Read the model definition and answer for the solid it produces. Units are mm, in the model's axes. A direction names the side the tool comes from. Coordinates: 2 decimals unless noted, no trailing zeros. Loops run counter-clockwise (first coordinate to the right, second up) from the corner with the lowest first, then second, coordinate; pieces in that order, holes last.
from build123d import *

# Parameters (mm, degrees)
SKETCH1_R           = 1.675
BOSS_EXTRUDE1_DEPTH = 4
CUT_EXTRUDE1_DEPTH  = 2.5
SKETCH3_R           = 1.6
BOSS_EXTRUDE2_DEPTH = 4.5
FILLET1_R           = 0.5


with BuildPart() as part:
    # Sketch1 → Boss-Extrude1 (new body, symmetric)
    with BuildSketch(Plane.XY):
        with BuildLine():
            Line((13, -4.031128874), (17, -4.031128874))
            ThreePointArc((17, -4.031128874), (15, 4.5), (13, -4.031128874))
        make_face()
        with Locations((15, 0)):
            Circle(SKETCH1_R, mode=Mode.SUBTRACT)
    extrude(amount=BOSS_EXTRUDE1_DEPTH, both=True)

    # Sketch2 → Cut-Extrude1 (cut, symmetric)
    with BuildSketch(Plane.XY):
        with BuildLine():
            Line((11.381384933, -2.675), (18.618615067, -2.675))
            ThreePointArc((18.618615067, -2.675), (15, 4.5), (11.381384933, -2.675))
        make_face()
    extrude(amount=CUT_EXTRUDE1_DEPTH, both=True, mode=Mode.SUBTRACT)

    # Sketch3 → Boss-Extrude2 (add)
    with BuildSketch(Plane.XZ.offset(4.031128874)):
        with Locations((15, 0)):
            Circle(SKETCH3_R)
    extrude(amount=BOSS_EXTRUDE2_DEPTH)

    # Fillet1
    fillet1_edges = [part.edges().sort_by_distance(p)[0] for p in [
        (13.4, -4.031128874, 0),
    ]]
    fillet(fillet1_edges, radius=FILLET1_R)


solid = part.part
Item 1: Which of the six approach directions +Z, -Z, +X, -X, +Y, -Y give full straight-line access (tool end or side, diameter ignored) to faces 5 (the face through (15, 2, -2.5)), 6 (the face through (17.97, -3.38, 0.06))?
Numbers:
face 5: +X, -X, +Y
face 6: +Z, -Z
Item 2: A cutting plane is placed at D-D on z = 2.25. Determine the outline of the cut face in (x, y) (3 decimals), then the cut area to 3 significant figures.
Numbers:
outline: (11.381, -2.675) arc R4.5 ccw to (13, -4.031) - (17, -4.031) arc R4.5 ccw to (18.619, -2.675) - close
area: 7.97 mm2
Item 3: A cutting plane is placed at B-B on x = 15. Determine the outline of the cut face in (y, z) (3 decimals), then the cut area to 3 significant figures.
Numbers:
outline: (-8.531, -1.6) - (-4.531, -1.6) arc R0.5 cw to (-4.031, -2.1) - (-4.031, -4) - (-1.675, -4) - (-1.675, -2.5) - (-2.675, -2.5) - (-2.675, 2.5) - (-1.675, 2.5) - (-1.675, 4) - (-4.031, 4) - (-4.031, 2.1) arc R0.5 cw to (-4.531, 1.6) - (-8.531, 1.6) - close; (1.675, -4) - (4.5, -4) - (4.5, -2.5) - (1.675, -2.5) - close; (1.675, 2.5) - (4.5, 2.5) - (4.5, 4) - (1.675, 4) - close
area: 36.8 mm2
Item 4: A cutting plane is placed at A-A on y = 0. Determine the outline of the cut face in (x, z) (3 decimals).
Numbers:
outline: (10.5, -4) - (13.325, -4) - (13.325, -2.5) - (10.5, -2.5) - close; (10.5, 2.5) - (13.325, 2.5) - (13.325, 4) - (10.5, 4) - close; (16.675, -4) - (19.5, -4) - (19.5, -2.5) - (16.675, -2.5) - close; (16.675, 2.5) - (19.5, 2.5) - (19.5, 4) - (16.675, 4) - close
Item 5: A cutting plane is placed at C-C on x = 11.75. Determine the outline of the cut face in (y, z) (3 decimals).
Numbers:
outline: (-3.112, -4) - (3.112, -4) - (3.112, -2.5) - (-2.675, -2.5) - (-2.675, 2.5) - (3.112, 2.5) - (3.112, 4) - (-3.112, 4) - close
Item 6: Given pin 1 (4.5 mm diameter, centred on x = 15, y = 0, fed in from -Z); pin 2 (1 mm diameter, centred on x = 15.5, z = -3, fed in from -Y); pin 3 (1 mm diameter, centred on x = 14, y = -6.5, fed in from +Z); pin 4 (3 mm diameter, centred on y = 2.5, z = -0.5, fed in from -X), each flat-ended and moving along its own axis, determine where each tip first touches the part or whether it passes through.
Numbers:
pin 1: stops at z = -4
pin 2: stops at y = -4.03
pin 3: stops at z = 1.52
pin 4: passes through
Item 7: Find the intervals of material crossed by line 1 along Y through (x, z) = (15, -3.55) (3 decimals); line 2 along Z through (x, y) = (18, -0.25); line 3 along X through (y, z) = (0, -3.35) (3 decimals), in increasing order.
Numbers:
line 1: y = -4.031 to -1.675, 1.675 to 4.5
line 2: z = -4 to -2.5, 2.5 to 4
line 3: x = 10.5 to 13.325, 16.675 to 19.5
Item 8: Determine the mould class of faces 1 (the face through (15, -2.675, 0)), 2 (the face through (14, -2, -4)), 3 (the face through (13.4, -6.5, 0.07)), 4 (the face through (15, 2, 2.5)) for opening direction Z: released by +Z, released by -Z, zero draft, split by the parting line, or undercut.
Numbers:
face 1: undercut
face 2: released by -Z
face 3: split by the parting line
face 4: undercut
